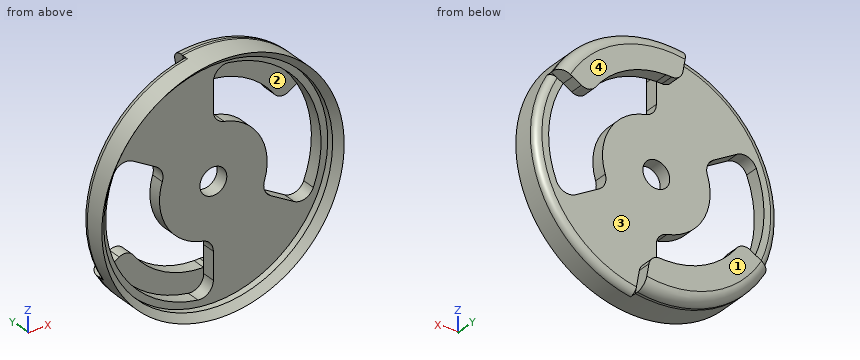
```python
from build123d import *

# Parameters (mm, degrees)
SKETCH_1_R          = 9
EXTRUDE_1_DEPTH     = 2
SKETCH_2_R          = 8.5
CUT_EXTRUDE_1_DEPTH = 1
CHAMFER_1_SIZE      = 0.5
CUT_EXTRUDE_2_DEPTH = 1
FILLET_1_R          = 1
SKETCH_4_R          = 1
CUT_EXTRUDE_3_DEPTH = 13.884098727
EXTRUDE_START       = 1
EXTRUDE_2_DEPTH     = 1
FILLET_3_R          = 0.8
FILLET_4_R          = 0.8
FILLET_5_R          = 0.5


# Some blends are built 0.0001 mm under size
with BuildPart() as part:
    # 草图1 → 凸台-拉伸1 (new body)
    with BuildSketch(Plane(origin=(0, 0, 0), x_dir=(1, 0, 0), z_dir=(0, 1, 0))):
        with Locations(Location((0, 0, 0), (0, 0, 270))):
            Circle(SKETCH_1_R)
    extrude(amount=EXTRUDE_1_DEPTH)

    # 草图2 → 切除-拉伸1 (cut)
    with BuildSketch(Plane.XZ):
        with Locations(Location((0, 0, 0), (0, 0, 270))):
            Circle(SKETCH_2_R)
    extrude(amount=-CUT_EXTRUDE_1_DEPTH, mode=Mode.SUBTRACT)

    # 倒角1
    chamfer_1_edges = [part.edges().sort_by_distance(p)[0] for p in [
        (0, 0, 8.5),
    ]]
    chamfer(chamfer_1_edges, length=CHAMFER_1_SIZE - 0.0001)  # a hair under: the kernel refuses the full size

    # 草图3 → 切除-拉伸2 (cut)
    with BuildSketch(Plane(origin=(0, 2, 0), x_dir=(1, 0, 0), z_dir=(0, 1, 0))):
        with BuildLine():
            Line((0, 4), (0, 8))
            ThreePointArc((0, 8), (-6.92820323, 4), (-6.92820323, -4))
            Line((-6.92820323, -4), (-3.464101615, -2))
            ThreePointArc((-3.464101615, -2), (-3.464101615, 2), (0, 4))
        make_face()
        with BuildLine():
            ThreePointArc((0, -8), (6.92820323, -4), (6.92820323, 4))
            Line((6.92820323, 4), (3.464101615, 2))
            ThreePointArc((3.464101615, 2), (3.464101615, -2), (0, -4))
            Line((0, -4), (0, -8))
        make_face()
    extrude(amount=-CUT_EXTRUDE_2_DEPTH, mode=Mode.SUBTRACT)

    # 圆角1
    fillet_1_edges = [part.edges().sort_by_distance(p)[0] for p in [
        (0, 1.5, -8),
        (0, 1.5, -4),
        (-3.464101615, 1.5, 2),
        (-6.92820323, 1.5, 4),
        (0, 1.5, 8),
        (0, 1.5, 4),
        (3.464101615, 1.5, -2),
        (6.92820323, 1.5, -4),
    ]]
    fillet(fillet_1_edges, radius=FILLET_1_R)

    # 草图4 → 切除-拉伸3 (cut, through all)
    with BuildSketch(Plane(origin=(0, 2, 0), x_dir=(1, 0, 0), z_dir=(0, 1, 0))):
        with Locations(Location((0, 0, 0), (0, 0, 270))):
            Circle(SKETCH_4_R)
    extrude(amount=-CUT_EXTRUDE_3_DEPTH, mode=Mode.SUBTRACT)

    # 草图5 → 凸台-拉伸2 (add)
    with BuildSketch(Plane(origin=(0, 2, 0), x_dir=(1, 0, 0), z_dir=(0, 1, 0)).offset(EXTRUDE_START)):
        with BuildLine():
            ThreePointArc((1.562833599, 8.863269777), (-3.803564356, 8.156770083), (-7.794228634, 4.5))
            Line((-7.794228634, 4.5), (-6.92820323, 4))
            ThreePointArc((-6.92820323, 4), (-4.485875631, 6.623965566), (-1.142857143, 7.917946549))
            ThreePointArc((-1.142857143, 7.917946549), (-0.345346329, 7.684132176), (0, 6.92820323))
            Line((0, 6.92820323), (0, 6.5))
            ThreePointArc((0, 6.5), (0.566512328, 6.475265538), (1.128713155, 6.401250395))
            Line((1.128713155, 6.401250395), (1.562833599, 8.863269777))
        make_face()
        with BuildLine():
            ThreePointArc((-1.142857143, 7.917946549), (-4.485875631, 6.623965566), (-6.92820323, 4))
            Line((-6.92820323, 4), (-5.629165125, 3.25))
            ThreePointArc((-5.629165125, 3.25), (-3.25, 5.629165125), (0, 6.5))
            Line((0, 6.5), (0, 6.92820323))
            ThreePointArc((0, 6.92820323), (-0.345346329, 7.684132176), (-1.142857143, 7.917946549))
        make_face()
        with BuildLine():
            ThreePointArc((5.629165125, -3.25), (3.25, -5.629165125), (0, -6.5))
            Line((0, -6.5), (0, -6.92820323))
            ThreePointArc((0, -6.92820323), (0.345346329, -7.684132176), (1.142857143, -7.917946549))
            ThreePointArc((1.142857143, -7.917946549), (4.485875631, -6.623965566), (6.92820323, -4))
            Line((6.92820323, -4), (5.629165125, -3.25))
        make_face()
        with BuildLine():
            Line((-1.128713155, -6.401250395), (-1.562833599, -8.863269777))
            ThreePointArc((-1.562833599, -8.863269777), (3.803564356, -8.156770083), (7.794228634, -4.5))
            Line((7.794228634, -4.5), (6.92820323, -4))
            ThreePointArc((6.92820323, -4), (4.485875631, -6.623965566), (1.142857143, -7.917946549))
            ThreePointArc((1.142857143, -7.917946549), (0.345346329, -7.684132176), (0, -6.92820323))
            Line((0, -6.92820323), (0, -6.5))
            ThreePointArc((0, -6.5), (-0.566512328, -6.475265538), (-1.128713155, -6.401250395))
        make_face()
    extrude(amount=-EXTRUDE_2_DEPTH)

    # 圆角3
    fillet_3_edges = [part.edges().sort_by_distance(p)[0] for p in [
        (-3.803564356, 3, -8.156770083),
        (3.803564356, 3, 8.156770083),
    ]]
    fillet(fillet_3_edges, radius=FILLET_3_R)

    # 圆角4
    fillet_4_edges = [part.edges().sort_by_distance(p)[0] for p in [
        (-5.629165125, 2.5, -3.25),
        (1.128713155, 2.5, -6.401250395),
        (5.629165125, 2.5, 3.25),
        (-1.128713155, 2.5, 6.401250395),
    ]]
    fillet(fillet_4_edges, radius=FILLET_4_R)

    # 圆角5
    # the kernel refuses this fillet: 0.5 mm, written as the material it takes off along each edge
    with BuildSketch(Plane(origin=(0, 2, 0), x_dir=(-0.8660254037844409, 0, -0.49999999999999595), z_dir=(0.49999999999999595, 0, -0.8660254037844409))) as fillet_5_piece_1:
        with BuildLine():
            CenterArc((9 - FILLET_5_R, -FILLET_5_R), FILLET_5_R, 0, 90)
            Line((9 - FILLET_5_R, 0), (9, 0))
            Line((9, 0), (9, -FILLET_5_R))
        make_face()
    revolve(axis=Axis((0, 2, 0), (0, 1, 0)), revolution_arc=110, mode=Mode.SUBTRACT)
    with BuildSketch(Plane(origin=(0, 2, 0), x_dir=(0.866025403784441, 0, 0.49999999999999584), z_dir=(-0.49999999999999584, 0, 0.866025403784441))) as fillet_5_piece_2:
        with BuildLine():
            CenterArc((9 - FILLET_5_R, -FILLET_5_R), FILLET_5_R, 0, 90)
            Line((9 - FILLET_5_R, 0), (9, 0))
            Line((9, 0), (9, -FILLET_5_R))
        make_face()
    revolve(axis=Axis((0, 2, 0), (0, 1, 0)), revolution_arc=110, mode=Mode.SUBTRACT)


solid = part.part
```
Geometry check sheet. Reference: the model listing, model coordinates, mm. Face numbers are marked on the shaded views. A direction names the side the tool comes from. Coordinates: 2 decimals unless noted, no trailing zeros. Write each loop counter-clockwise with the first axis right and the second up, starting at its lowest first coordinate (ties: lowest second). Pieces come first, ordered by that corner, then holes. Notation, with made-up numbers: M 14,-9 L 59,-9 A11 cw 59,-1 Z; hole C -21.5,3.5 d7. An arc over 180 degrees is marked long. Use one line per item in the form item = value. Start each with the question number.
1) Section check B-B on y = 2.55. Enter the section's corners in (x, z), and give its area (3 significant figures).
2) Set-up check for the marked faces 1 and 2: record each of +Z, -Z, +X, -X, +Y, -Y from which the full face is reachable in a straight line by a thin tool's end or side.
3) Thickness scan on probe 1 along X at (y, z) = (1.4, 0); probe 2 along X at (y, z) = (0.7, 0); probe 3 along X at (y, z) = (1.45, 1.75). Record the ranges inside material, lowest first. Write a range as from..to.
4) Go/stop test with flat-tipped pins: pin 1 Ø0.5 at (y, z) = (1.5, 6) entering from +X; pin 2 Ø5 at (x, z) = (0.5, -1.5) entering from +Y; pin 3 Ø0.5 at (y, z) = (1.5, -6.5) entering from -X. Record where each tip stops, or that it passes through.
5) Section check A-A on z = 0. State how many separate pieces and enclosed holes the cut face has, and give its area (3 significant figures).
6) Release check for a two-part mould opening along Z. For the marked faces 3 and 4 record: pulls with the +Z half, pulls with the -Z half, needs draft (parallel to the pull), parting line crosses it, or undercut.
Responses:
q1.outline = M -7.72,-4.46 A8.92 ccw 1.55,-8.78 L 1.26,-7.15 A0.8 ccw 0.42,-6.49 A6.5 cw -5.24,-3.85 A0.8 ccw -6.28,-3.63 Z; M -1.55,8.78 L -1.26,7.15 A0.8 ccw -0.42,6.49 A6.5 cw 5.24,3.85 A0.8 ccw 6.28,3.63 L 7.72,4.46 A8.92 ccw Z
q1.area = 45.1 mm2
q2.face_1 = +Z, -Z, +X, -X, +Y
q2.face_2 = -Y
q3.probe_1 = -9..-8, -4..-1, 1..4, 8..9
q3.probe_2 = -9..-8.5, 8.5..9
q3.probe_3 = -8.83..-7.81, -3.76..3.6, 7.81..8.83
q4.pin_1 = 6.92
q4.pin_2 = 2
q4.pin_3 = -6.48
q5.separate_pieces = 4
q5.enclosed_holes = 0
q5.area = 8.64 mm2
q6.face_3 = undercut
q6.face_4 = needs draft
